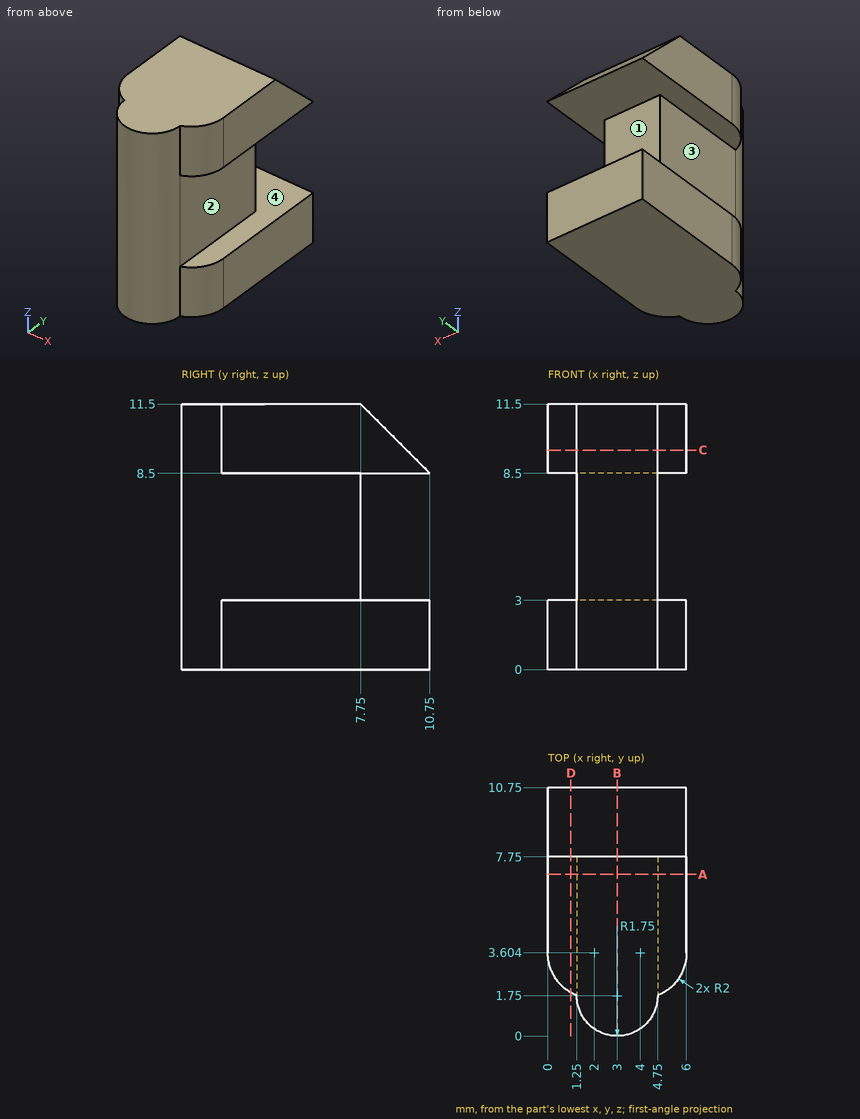
Could you check a few things on this drawing? It's one solid part, dimensions in mm from its lowest x, y, z. A direction names the side the tool comes from. Round coordinates to 2 decimals unless told otherwise and drop trailing zeros. Write each loop counter-clockwise with the first axis right and the second up, starting at its lowest first coordinate (ties: lowest second). Pieces come first, ordered by that corner, then holes. Notation, with made-up numbers: (71.5, -37.5) -> (77.5, -37.5) arc R26 ccw to (77.5, -14.5) -> close; hole circle Ø7 at (79.5, 77). An arc over 180 degrees is marked (long way). Use one line per item in the form item = value. Start each with the question number.
Q1. If I drill on probe 1 along Z at (x, y) = (5.5, 8.25); probe 2 along X at (y, z) = (5.5, 3.5); probe 3 along Z at (x, y) = (1.75, 8.75), over which ranges is the centre line in solid material (lowest first)? Write a range as [from, to].
Q2. Imagine slicing it at C-C (z = 9.5). Please give me the cut outline in (x, y).
Q3. Imagine slicing it at B-B (x = 3). Please give me the cut outline in (y, z), then the cut area to 3 significant figures.
Q4. I'm going to push flat-ended pins straight in: P1, Ø1.6, axis at y = 5.5, z = 6.5, coming from the -X side; P2, Ø1, axis at x = 1.5, z = 1.5, coming from the -Y side; P3, Ø4.5, axis at y = 5, z = 6, coming from the +X side. Where does each tip first touch, or does it pass through?
Q5. Which directions (+Z, -Z, +X, -X, +Y, -Y) give clear straight access to the entire face, cutting with the end or side of a thin tool? Please do the marked faces 1, 2, 3 and 4.
Q6. Imagine slicing it at D-D (x = 1). Please give me the cut outline in (y, z), then the cut area to 3 significant figures.
Q7. Imagine slicing it at A-A (y = 7). Please give me the cut outline in (x, z).
Worked out:
q1.probe_1 = [0, 3], [8.5, 11]
q1.probe_2 = [1.25, 4.75]
q1.probe_3 = [0, 3], [8.5, 10.5]
q2.outline = (0, 3.6) arc R2 ccw to (1.25, 1.75) arc R1.75 ccw to (4.75, 1.75) arc R2 ccw to (6, 3.6) -> (6, 9.75) -> (0, 9.75) -> close
q3.outline = (0, 0) -> (10.75, 0) -> (10.75, 3) -> (7.75, 3) -> (7.75, 8.5) -> (10.75, 8.5) -> (7.75, 11.5) -> (0, 11.5) -> close
q3.area = 103 mm^2
q4.P1 = 1.25
q4.P2 = 0.31
q4.P3 = 4.75
q5.face_1 = +X, -X, +Y
q5.face_2 = +X, +Y, -Y
q5.face_3 = -X, +Y, -Y
q5.face_4 = +Y
q6.outline = (1.87, 0) -> (10.75, 0) -> (10.75, 3) -> (1.87, 3) -> close; (1.87, 8.5) -> (10.75, 8.5) -> (7.75, 11.5) -> (1.87, 11.5) -> close
q6.area = 48.8 mm^2
q7.outline = (0, 0) -> (6, 0) -> (6, 3) -> (4.75, 3) -> (4.75, 8.5) -> (6, 8.5) -> (6, 11.5) -> (0, 11.5) -> (0, 8.5) -> (1.25, 8.5) -> (1.25, 3) -> (0, 3) -> close
